```python
from build123d import *

# Parameters (mm, degrees)
F1_DEPTH             = 96
F3_DEPTH             = 40.001
F6_D                 = 3.3
F6_DEPTH             = 30
F6_CBORE_D           = 6.5
F6_CBORE_DEPTH       = 3
F6_TIP               = 0.9914200214
F6_ON_F4_D           = 3.3
F6_ON_F4_DEPTH       = 30
F6_ON_F4_CBORE_D     = 6.5
F6_ON_F4_CBORE_DEPTH = 3
F6_ON_F4_TIP         = 0.9914200214
F8_DEPTH             = 40.001
F10_DEPTH            = 3
F12_DEPTH            = 3
F14_DEPTH            = 3
F15_W                = 40
F15_H                = 8
F16_DEPTH            = 2
F17_R                = 1.65
F18_DEPTH            = 8
F20_SIZE             = 4
F22_DEPTH            = 64.001
F23_R                = 1.65
F24_DEPTH            = 25


with BuildPart() as f1:
    # F0 (on Front) → F1 (new body)
    with BuildSketch(Plane.XZ):
        with BuildLine():
            Line((0, 24), (0, 0))
            Line((0, 0), (40, 0))
            Line((40, 0), (40, 24))
            Line((40, 24), (31.0797111876, 24))
            ThreePointArc((31.0797111876, 24), (20, 17.4), (8.9202888124, 24))
            Line((8.9202888124, 24), (0, 24))
        make_face()
    extrude(amount=F1_DEPTH)

    # F2 (on face) → F3 (cut, through all)
    with BuildSketch(Plane.YZ.offset(40)):
        with BuildLine():
            Line((-87.25, 0), (-87.25, 8.0709415886))
            ThreePointArc((-87.25, 8.0709415886), (-88, 16), (-88.75, 8.0709415886))
            Line((-88.75, 8.0709415886), (-88.75, 0))
            Line((-88.75, 0), (-87.25, 0))
        make_face()
        with BuildLine():
            Line((-7.25, 0), (-7.25, 8.0709415886))
            ThreePointArc((-7.25, 8.0709415886), (-8, 16), (-8.75, 8.0709415886))
            Line((-8.75, 8.0709415886), (-8.75, 0))
            Line((-8.75, 0), (-7.25, 0))
        make_face()
    extrude(amount=-F3_DEPTH, mode=Mode.SUBTRACT)

    # F6
    with Locations(Plane.XZ.offset(96)):
        with Locations((8, 5), (32, 5)):
            CounterBoreHole(F6_D / 2, F6_CBORE_D / 2, F6_CBORE_DEPTH, depth=F6_DEPTH)
            with Locations((0, 0, -(F6_DEPTH + F6_TIP / 2))):  # 118° drill point
                Cone(0, F6_D / 2, F6_TIP, mode=Mode.SUBTRACT)

    # F6 on F4
    with Locations(Plane(origin=(0, 0, 0), x_dir=(-1, 0, 0), z_dir=(0, 1, 0))):
        with Locations((-8, 5), (-32, 5)):
            CounterBoreHole(F6_ON_F4_D / 2, F6_ON_F4_CBORE_D / 2, F6_ON_F4_CBORE_DEPTH, depth=F6_ON_F4_DEPTH)
            with Locations((0, 0, -(F6_ON_F4_DEPTH + F6_ON_F4_TIP / 2))):  # 118° drill point
                Cone(0, F6_ON_F4_D / 2, F6_ON_F4_TIP, mode=Mode.SUBTRACT)

    # F7 (on face) → F8 (cut, through all)
    with BuildSketch(Plane(origin=(0, 0, 0), x_dir=(0, -1, 0), z_dir=(-1, 0, 0))):
        with BuildLine():
            Line((18, 11), (18, 0))
            Line((18, 0), (78, 0))
            Line((78, 0), (78, 11))
            ThreePointArc((78, 11), (76.5355339059, 14.5355339059), (73, 16))
            Line((73, 16), (23, 16))
            ThreePointArc((23, 16), (19.4644660941, 14.5355339059), (18, 11))
        make_face()
    extrude(amount=-F8_DEPTH, mode=Mode.SUBTRACT)

    # F9 (on face) → F10 (cut)
    with BuildSketch(Plane(origin=(0, 0, 16), x_dir=(1, 0, 0), z_dir=(0, 0, -1))):
        Polygon((7.5, 66.2679491924), (7.5, 69.7320508076), (4.5, 71.4641016151), (1.5, 69.7320508076), (1.5, 66.2679491924), (4.5, 64.5358983849), align=None)
        Polygon((32.5, 69.7320508076), (32.5, 66.2679491924), (35.5, 64.5358983849), (38.5, 66.2679491924), (38.5, 69.7320508076), (35.5, 71.4641016151), align=None)
        Polygon((7.5, 26.2679491924), (7.5, 29.7320508076), (4.5, 31.4641016151), (1.5, 29.7320508076), (1.5, 26.2679491924), (4.5, 24.5358983849), align=None)
        Polygon((32.5, 29.7320508076), (32.5, 26.2679491924), (35.5, 24.5358983849), (38.5, 26.2679491924), (38.5, 29.7320508076), (35.5, 31.4641016151), align=None)
    extrude(amount=-F10_DEPTH, mode=Mode.SUBTRACT)

    # F11 (on face) → F12 (cut)
    with BuildSketch(Plane.XZ.offset(18)):
        Polygon((11, 3.2679491924), (11, 6.7320508076), (8, 8.4641016151), (5, 6.7320508076), (5, 3.2679491924), (8, 1.5358983849), align=None)
        Polygon((35, 3.2679491924), (35, 6.7320508076), (32, 8.4641016151), (29, 6.7320508076), (29, 3.2679491924), (32, 1.5358983849), align=None)
    extrude(amount=-F12_DEPTH, mode=Mode.SUBTRACT)

    # F13 (on face) → F14 (cut)
    with BuildSketch(Plane(origin=(0, -78, 0), x_dir=(-1, 0, 0), z_dir=(0, 1, 0))):
        Polygon((-35, 6.7320508076), (-35, 3.2679491924), (-32, 1.5358983849), (-29, 3.2679491924), (-29, 6.7320508076), (-32, 8.4641016151), align=None)
        Polygon((-11, 6.7320508076), (-11, 3.2679491924), (-8, 1.5358983849), (-5, 3.2679491924), (-5, 6.7320508076), (-8, 8.4641016151), align=None)
    extrude(amount=-F14_DEPTH, mode=Mode.SUBTRACT)

    # F15 (on face) → F16 (join)
    with BuildSketch(Plane(origin=(0, 0, 16), x_dir=(1, 0, 0), z_dir=(0, 0, -1))):
        with Locations((20, 36)):
            Rectangle(F15_W, F15_H)
    extrude(amount=F16_DEPTH)


with BuildPart() as f18:
    # F17 (on face) → F18 (new body)
    with BuildSketch(Plane.XZ.offset(40)):
        with BuildLine():
            Line((40, -28.2), (40, 14))
            Line((40, 14), (-2.2, 14))
            Line((-2.2, 14), (-2.2, 3.9))
            Line((-2.2, 3.9), (18.9, 3.9))
            ThreePointArc((18.9, 3.9), (29.9, -7.1), (18.9, -18.1))
            Line((18.9, -18.1), (-2.2, -18.1))
            Line((-2.2, -18.1), (-2.2, -28.2))
            Line((-2.2, -28.2), (40, -28.2))
        make_face()
        with Locations((3.4, -22.6)):
            Circle(F17_R, mode=Mode.SUBTRACT)
        with Locations((34.4, -22.6)):
            Circle(F17_R, mode=Mode.SUBTRACT)
        with Locations((3.4, 8.4)):
            Circle(F17_R, mode=Mode.SUBTRACT)
        with Locations((34.4, 8.4)):
            Circle(F17_R, mode=Mode.SUBTRACT)
    extrude(amount=-F18_DEPTH)


with BuildPart() as f1_1:
    add(f1.part)

    # F19: union F18
    add(f18.part)

    # F20
    f20_edges = [f1_1.edges().sort_by_distance(p)[0] for p in [
        (-2.2, -36, -28.2),
        (40, -36, -28.2),
    ]]
    chamfer(f20_edges, length=F20_SIZE)

    # F21 (on face) → F22 (cut, through all)
    with BuildSketch(Plane(origin=(0, -32, 0), x_dir=(-1, 0, 0), z_dir=(0, 1, 0))):
        Polygon((0, 15), (0, 14), (0, 12.2), (2.2, 10), (3.2, 10), (3.2, 15), align=None)
    extrude(amount=-F22_DEPTH, mode=Mode.SUBTRACT)

    # F23 (on face) → F24 (cut)
    with BuildSketch(Plane(origin=(0, 0, 16), x_dir=(1, 0, 0), z_dir=(0, 0, -1))):
        with Locations((35.5, 68)):
            Circle(F23_R)
        with Locations((4.5, 68)):
            Circle(F23_R)
        with Locations((35.5, 28)):
            Circle(F23_R)
        with Locations((4.5, 28)):
            Circle(F23_R)
    extrude(amount=-F24_DEPTH, mode=Mode.SUBTRACT)


solid = f1_1.part
```
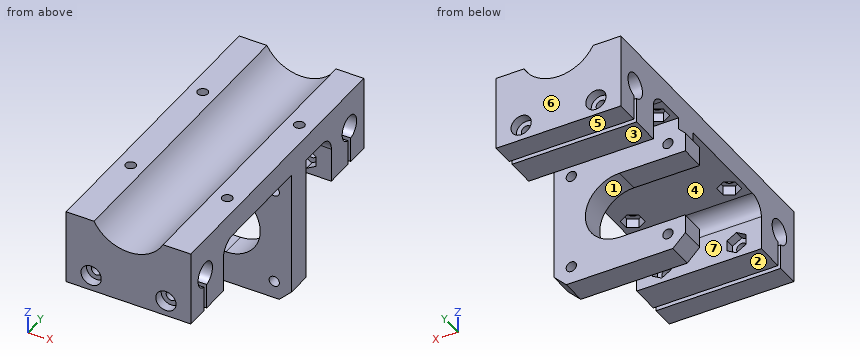
Check sheet for the modelled part. Datum: model origin and axes. Units: mm. Face numbers are marked on the shaded views. A direction names the side the tool comes from. Coordinates: 2 decimals unless noted, no trailing zeros. Order: outer loops, then holes, each group sorted by start corner. A loop starts at its lowest first (then second) coordinate and runs counter-clockwise, first axis right, second up. Notation, with made-up numbers: (59, 16) -> (96, 16) arc R27 ccw to (96, 47) -> close; hole circle Ø5 at (47.5, 5.5). An arc over 180 degrees is marked (long way). Write item = value, one per line. Start each with the question number.
1) Material ranges on L1, parallel to Y at x = 26, z = 2.5; L2, parallel to Z at x = 32, y = -13; L3, parallel to Z at x = 7, y = -35, recorded low to high.
2) Cross-section at A-A (y = -68). Enter the section's corners in (x, z), then the cut area to 3 significant figures.
3) Cross-section at D-D (y = -5.5). Enter the section's corners in (x, z), then the cut area to 3 significant figures.
4) Go/stop test with flat-tipped pins: P1, Ø7, axis at x = 21.5, y = -26.5, coming from the -Z side; P2, Ø6.5, axis at x = 31, z = 6, coming from the -Y side; P3, Ø2, axis at x = 20.5, y = -92, coming from the -Z side; P4, Ø4, axis at x = 32, z = 5, coming from the -Y side. Record where each tip stops, or that it passes through.
5) Access from +Z, -Z, +X, -X, +Y, -Y to the whole of each face (thin tool, end or side, straight path). Record for the marked faces 1, 2, 3 and 4.
6) Cross-section at C-C (z = 20). Enter the section's corners in (x, y).
7) Cross-section at B-B (x = 14.5). Enter the section's corners in (y, z), then the cut area to 3 significant figures.
8) Mould release check, pull along Y, two halves, no side actions. Record for the marked faces 5, 6 and 7: +Y half, -Y half, draft (parallel to the pull), parting line (faces both ways), or undercut.
Ans:
q1.L1 = -96 to -88.75, -87.25 to -78, -40 to -32, -18 to -8.75, -7.25 to 0
q1.L2 = 0 to 3.35, 6.65 to 24
q1.L3 = -28.2 to -18.1, 3.9 to 24
q2.outline = (0, 16) -> (1.5, 16) -> (1.5, 19) -> (2.85, 19) -> (2.85, 24) -> (0, 24) -> close; (6.15, 19) -> (7.5, 19) -> (7.5, 16) -> (32.5, 16) -> (32.5, 19) -> (33.85, 19) -> (33.85, 24) -> (31.08, 24) arc R12.6 cw to (8.92, 24) -> (6.15, 24) -> close; (37.15, 19) -> (38.5, 19) -> (38.5, 16) -> (40, 16) -> (40, 24) -> (37.15, 24) -> close
q2.area = 147 mm²
q3.outline = (0, 0) -> (40, 0) -> (40, 8.88) -> (0, 8.88) -> close; (0, 15.12) -> (40, 15.12) -> (40, 24) -> (31.08, 24) arc R12.6 cw to (8.92, 24) -> (0, 24) -> close; hole circle Ø3.3 at (8, 5); hole circle Ø3.3 at (32, 5)
q3.area = 589 mm²
q4.P1 = 16
q4.P2 = -96
q4.P3 = 0
q4.P4 = -93
q5.face_1 = -X
q5.face_2 = -Z, +X, -X, -Y
q5.face_3 = -Z, +X, -X, +Y
q5.face_4 = -Z, +X, -X
q6.outline = (0, -96) -> (12.33, -96) -> (12.33, 0) -> (0, 0) -> close; (27.67, -96) -> (40, -96) -> (40, 0) -> (27.67, 0) -> close; hole circle Ø3.3 at (4.5, -68); hole circle Ø3.3 at (4.5, -28); hole circle Ø3.3 at (35.5, -68); hole circle Ø3.3 at (35.5, -28)
q7.outline = (-96, 0) -> (-88.75, 0) -> (-88.75, 8.07) arc R4 cw (long way) to (-87.25, 8.07) -> (-87.25, 0) -> (-78, 0) -> (-78, 11) arc R5 cw to (-73, 16) -> (-40, 16) -> (-40, 3.9) -> (-32, 3.9) -> (-32, 16) -> (-23, 16) arc R5 cw to (-18, 11) -> (-18, 0) -> (-8.75, 0) -> (-8.75, 8.07) arc R4 cw (long way) to (-7.25, 8.07) -> (-7.25, 0) -> (0, 0) -> (0, 18.66) -> (-96, 18.66) -> close; (-40, -28.2) -> (-32, -28.2) -> (-32, -18.1) -> (-40, -18.1) -> close
q7.area = 895 mm²
q8.face_5 = draft
q8.face_6 = +Y half
q8.face_7 = undercut
